from build123d import *

# Parameters (mm, degrees)
REVOLVE1_ANGLE     = 180
SKETCH3_R          = 12.5
SPOT1_DEPTH        = 10
SKETCH4_R          = 12.5
SPOT2_DEPTH        = 10
SKETCH6_R          = 12.5
SPOT3_DEPTH        = 10
SKETCH7_W          = 8.5
SKETCH7_H          = 12.7
CUT_EXTRUDE4_DEPTH = 107


with BuildPart() as part:
    # Sketch1 → Revolve1 (revolve)
    with BuildSketch(Plane.XY):
        with BuildLine():
            Line((-106, 0), (-100, 0))
            ThreePointArc((-100, 0), (-84.638501094, 26.186146828), (-54.285714286, 25.5550626))
            ThreePointArc((-54.285714286, 25.5550626), (13.093073414, 58.554004377), (60, 0))
            Line((60, 0), (66, 0))
            ThreePointArc((66, 0), (17.369924747, 63.673273155), (-56.857142857, 33.515150397))
            ThreePointArc((-56.857142857, 33.515150397), (-90.283702113, 29.741745554), (-106, 0))
        make_face()
    revolve(axis=Axis((-106, 0, 0), (1, 0, 0)), revolution_arc=REVOLVE1_ANGLE)

    # Sketch3 → Spot1 (cut)
    with BuildSketch(Plane(origin=(-35.461774151, 27.831917712, 48.206295549), x_dir=(0.833827643, 0.395653782, 0.384953954), z_dir=(-0.537299608, 0.421695723, 0.730398417))):
        Circle(SKETCH3_R)
    spot1 = extrude(amount=-SPOT1_DEPTH, mode=Mode.SUBTRACT)

    # Sketch4 → Spot2 (cut)
    with BuildSketch(Plane(origin=(35.461774151, 27.831917712, 48.206295549), x_dir=(0.843391446, -0.268649804, -0.46531511), z_dir=(0.537299608, 0.421695723, 0.730398417))):
        Circle(SKETCH4_R)
    spot2 = extrude(amount=-SPOT2_DEPTH, mode=Mode.SUBTRACT)

    # Sketch6 → Spot3 (cut)
    with BuildSketch(Plane(origin=(0, 57.15767665, 33), x_dir=(1, 0, 0), z_dir=(0, 0.866025404, 0.5))):
        Circle(SKETCH6_R)
    spot3 = extrude(amount=-SPOT3_DEPTH, mode=Mode.SUBTRACT)

    # Mirror1: Spot1, Spot2, Spot3 across plane
    add(spot1.mirror(Plane.ZX), mode=Mode.SUBTRACT)
    add(spot2.mirror(Plane.ZX), mode=Mode.SUBTRACT)
    add(spot3.mirror(Plane.ZX), mode=Mode.SUBTRACT)

    # Sketch7 → Cut-Extrude4 (cut, through all)
    with BuildSketch(Plane(origin=(0, 0, 0), x_dir=(0, 0, -1), z_dir=(1, 0, 0))):
        with Locations((-4.25, 0)):
            Rectangle(SKETCH7_W, SKETCH7_H)
    extrude(amount=-CUT_EXTRUDE4_DEPTH, mode=Mode.SUBTRACT)


solid = part.part
Here's how the part is built. I have some questions about the finished solid (model axes, mm). A direction names the side the tool comes from. Give positions to 0.01 mm unless a question says otherwise; leave off trailing zeros. Order: outer loops, then holes, each group sorted by start corner. A loop starts at its lowest first (then second) coordinate and runs counter-clockwise, first axis right, second up. Notation, with made-up numbers: M 74.5,59 L 80.5,59 A22 ccw 80.5,82 Z; hole C -19,36 d1. An arc over 180 degrees is marked long. Answer as a JSON object with one key per item and string values. Group by question number.
1) On a 3-axis mill with a long thin cutter (end or side, diameter ignored), from which of +Z, -Z, +X, -X, +Y, -Y can I reach the whole of each face in a straight line? I mean faces 1 (the cylindrical face through (5.8, -48, 40.5)), 2 (the flat face through (-101, 0, 8.5)). Say none if no direction works.
2) Suppose I cut it at D-D, the plane x = 48. Write out the boundary of the cut face in (y, z), plus the area to 3 significant figures.
3) I'm going to push flat-ended pins straight in: pin 1 Ø10 at (x, z) = (-55.5, 11) entering from -Y; pin 2 Ø8 at (x, z) = (-103.5, 3.5) entering from -Y; pin 3 Ø1.5 at (y, z) = (23, 54) entering from -X; pin 4 Ø1.5 at (x, y) = (26, -32) entering from -Z. Where does each tip first touch, or does it pass through?
4) Suppose I cut it at C-C, the plane x = -78. Write out the boundary of the cut face in (y, z).
5) Suppose I cut it at A-A, the plane y = 3. Write out the boundary of the cut face in (x, z).
6) We'd pull the mould along X, two halves only. Please class faces 3 (the cylindrical face through (-26.984, -19.29, 53.607)), 4 (the flat face through (-102, 6.35, 4)): pulls with the +X half, pulls with the -X half, needs draft (parallel to the pull), parting line crosses it, or undercut.
7) Suppose I cut it at B-B, the plane z = 10.5. Write out the boundary of the cut face in (x, y).
8) Please list where these lines run through material, in increasing order: L1, parallel to X at y = -7.5, z = 15; L2, parallel to Y at x = -5.5, z = 8; L3, parallel to Y at x = -76, z = 20. Write a range as [from, to].
Results found:
{
 "1": {"face 1": "none", "face 2": "-Z, -X"},
 "2": {"outline": "M -45.3,0 L -36,0 A36 cw 36,0 L 45.3,0 A45.3 ccw Z", "area": "1,190 mm²"},
 "3": {"pin 1": "y = -41.18", "pin 2": "y = -20.37", "pin 3": "x = -25.71", "pin 4": "through"},
 "4": {"outline": "M -35.1,0 L -28.91,0 A28.91 cw 28.91,0 L 35.1,0 A35.1 ccw Z"},
 "5": {"outline": "M -104.85,8.5 L -98.61,8.5 A29.85 cw -54.29,25.38 A59.92 cw 59.92,0 L 65.93,0 A65.93 ccw -56.86,33.38 A35.87 ccw Z"},
 "6": {"face 3": "undercut", "face 4": "needs draft"},
 "7": {"outline": "M -56.86,-31.83 A65.16 ccw long -56.86,31.83 A34.43 ccw long Z; hole M -54.29,-23.3 A59.07 ccw long -54.29,23.3 A28.1 ccw long Z"},
 "8": {"L1": "[-101.86, -94.87], [57.61, 63.83]", "L2": "[-65.28, -59.21], [59.21, 65.28]", "L3": "[-29.33, -21.54], [21.54, 29.33]"}
}
